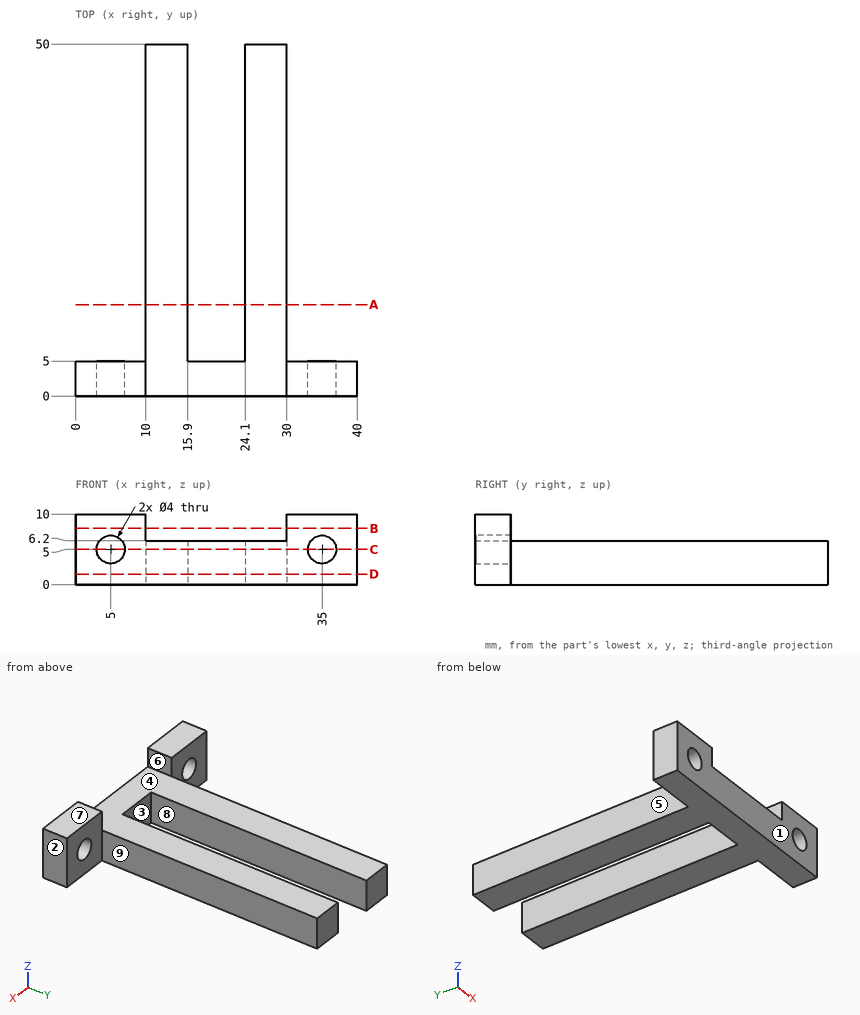
The drawing under review shows one solid part. Ordinate dimensions are in mm from its lowest x, y, z. A direction names the side the tool comes from. Give positions to 0.01 mm unless a question says otherwise; leave off trailing zeros. Order: outer loops, then holes, each group sorted by start corner. A loop starts at its lowest first (then second) coordinate and runs counter-clockwise, first axis right, second up. Notation, with made-up numbers: M -39,28 L -8,28 A24 cw -8,52 Z; hole C -6.75,12 d10. An arc over 180 degrees is marked long. One line per question, with ' | ' between items. Start each with the question number.
Q1. The part is to be moulded in two halves that separate along X. For the marked faces 1, 2, 3 and 4, say which applies: +X half, -X half, draft (parallel to the pull), parting line (faces both ways), or undercut.
Q2. We need section B-B (z = 8). Write out the cut boundary in (x, y), plus the area to 3 significant figures.
Q3. For pin 1 Ø3 at (y, z) = (35, 3.5) entering from +X; pin 2 Ø22 at (x, y) = (18.5, 24.5) entering from +Z; pin 3 Ø3 at (y, z) = (12, 7.5) entering from -X; pin 4 Ø1.5 at (y, z) = (22, 7) entering from -X, all flat-tipped, find the tip position at first contact; note any pin that passes through.
Q4. We need section A-A (y = 13). Write out the cut boundary in (x, z).
Q5. For L1, parallel to X at y = 1.5, z = 5; L2, parallel to X at y = 31.5, z = 5; L3, parallel to Y at x = 33.5, z = 8.75, list the stretches that pass through material, from the lowest coordinate up. Write a range as [from, to].
Q6. Machinability: for the marked faces 5, 6, 7, 8 and 9, which of the approach directions +Z, -Z, +X, -X, +Y, -Y give a long, thin tool a straight path to every point of the face, cutting with its end or side? Answer none if there is none.
Q7. We need section D-D (z = 1.5). Write out the cut boundary in (x, y).
Q8. We need section C-C (z = 5). Write out the cut boundary in (x, y), plus the area to 3 significant figures.
Returned:
1) face 1: draft | face 2: +X half | face 3: undercut | face 4: undercut
2) outline: M 0,0 L 10,0 L 10,5 L 0,5 Z; M 30,0 L 40,0 L 40,5 L 30,5 Z | area: 100 mm2
3) pin 1: x = 30 | pin 2: z = 6.2 | pin 3: x = 10 | pin 4: through
4) outline: M 10,0 L 15.9,0 L 15.9,6.2 L 10,6.2 Z; M 24.1,0 L 30,0 L 30,6.2 L 24.1,6.2 Z
5) L1: [0, 3], [7, 33], [37, 40] | L2: [10, 15.9], [24.1, 30] | L3: [0, 5]
6) face 5: +Z, -Z, -X, +Y | face 6: +Z, +Y, -Y | face 7: +Z, +X, -X, +Y, -Y | face 8: +Z, -Z, +Y | face 9: +Z, -Z, +X, +Y
7) outline: M 0,0 L 40,0 L 40,5 L 30,5 L 30,50 L 24.1,50 L 24.1,5 L 15.9,5 L 15.9,50 L 10,50 L 10,5 L 0,5 Z
8) outline: M 0,0 L 3,0 L 3,5 L 0,5 Z; M 7,0 L 33,0 L 33,5 L 30,5 L 30,50 L 24.1,50 L 24.1,5 L 15.9,5 L 15.9,50 L 10,50 L 10,5 L 7,5 Z; M 37,0 L 40,0 L 40,5 L 37,5 Z | area: 691 mm2
